Source: CAD feature listing. Evaluate the final solid. Frame: model axes, mm. Face numbers are marked on the shaded views. A direction names the side the tool comes from. Give positions to 0.01 mm unless a question says otherwise; leave off trailing zeros. Loops run counter-clockwise (first coordinate to the right, second up) from the corner with the lowest first, then second, coordinate; pieces in that order, holes last.
from build123d import *

# Parameters (mm, degrees)
SKETCH1_R                = 18.5
BOSS_EXTRUDE1_DEPTH      = 27.8
SKETCH2_R                = 17.1
BOSS_EXTRUDE2_DEPTH      = 25.2
SKETCH3_R                = 3.75
BOSS_EXTRUDE3_DEPTH      = 3.3
SKETCH4_R                = 6
BOSS_EXTRUDE4_DEPTH      = 6
SKETCH5_R                = 3
BOSS_EXTRUDE6_DEPTH      = 15
CUT_EXTRUDE1_START       = -12
CUT_EXTRUDE1_DEPTH       = 12
CUT_EXTRUDE2_DEPTH       = 1
M3_CLEARANCE_HOLE1_D     = 3.4
M3_CLEARANCE_HOLE1_DEPTH = 6
M3_CLEARANCE_HOLE1_TIP   = 1.021463052
SKETCH11_W               = 3
SKETCH11_H               = 0.5
BOSS_EXTRUDE7_DEPTH      = 8
FILLET1_R                = 1
CUT_EXTRUDE3_DEPTH       = 28


with BuildPart() as part:
    # Sketch1 → Boss-Extrude1 (new body)
    with BuildSketch(Plane.XY):
        Circle(SKETCH1_R)
    extrude(amount=BOSS_EXTRUDE1_DEPTH)

    # Sketch2 → Boss-Extrude2 (add)
    with BuildSketch(Plane(origin=(0, 0, 0), x_dir=(-1, 0, 0), z_dir=(0, 0, -1))):
        with Locations(Location((0, 0, 0), (0, 0, 180))):
            Circle(SKETCH2_R)
    extrude(amount=BOSS_EXTRUDE2_DEPTH)

    # Sketch3 → Boss-Extrude3 (add)
    with BuildSketch(Plane(origin=(0, 0, -25.2), x_dir=(-1, 0, 0), z_dir=(0, 0, -1))):
        Circle(SKETCH3_R)
    extrude(amount=BOSS_EXTRUDE3_DEPTH)

    # Sketch4 → Boss-Extrude4 (add)
    with BuildSketch(Plane.XY.offset(27.8)):
        with Locations((0, 7)):
            Circle(SKETCH4_R)
    extrude(amount=BOSS_EXTRUDE4_DEPTH)

    # Sketch5 → Boss-Extrude6 (add)
    with BuildSketch(Plane.XY.offset(33.8)):
        with Locations((0, 7)):
            Circle(SKETCH5_R)
    extrude(amount=BOSS_EXTRUDE6_DEPTH)

    # Sketch7 → Cut-Extrude1 (cut)
    with BuildSketch(Plane.XY.offset(48.8).offset(CUT_EXTRUDE1_START)):
        with BuildLine():
            Line((-1.8, 9.4), (1.8, 9.4))
            ThreePointArc((1.8, 9.4), (0, 10), (-1.8, 9.4))
        make_face()
    extrude(amount=CUT_EXTRUDE1_DEPTH, mode=Mode.SUBTRACT)

    # Sketch8 → Cut-Extrude2 (cut)
    with BuildSketch(Plane.XY.offset(27.8)):
        with BuildLine():
            ThreePointArc((8.923344727, 8.172142857), (0, -12.1), (-8.923344727, 8.172142857))
            ThreePointArc((-8.923344727, 8.172142857), (0, -2), (8.923344727, 8.172142857))
        make_face()
    extrude(amount=-CUT_EXTRUDE2_DEPTH, mode=Mode.SUBTRACT)

    # M3 Clearance Hole1
    with Locations(Plane.XY.offset(27.8)):
        with Locations((7.65, -13.250188678), (-7.65, -13.250188678), (-15.3, 0), (-7.65, 13.250188678), (15.3, 0), (7.65, 13.250188678)):
            Hole(M3_CLEARANCE_HOLE1_D / 2, depth=M3_CLEARANCE_HOLE1_DEPTH)
            with Locations((0, 0, -(M3_CLEARANCE_HOLE1_DEPTH + M3_CLEARANCE_HOLE1_TIP / 2))):  # 118° drill point
                Cone(0, M3_CLEARANCE_HOLE1_D / 2, M3_CLEARANCE_HOLE1_TIP, mode=Mode.SUBTRACT)

    # Sketch11 → Boss-Extrude7 (add)
    with BuildSketch(Plane(origin=(0, 0, -25.2), x_dir=(-1, 0, 0), z_dir=(0, 0, -1))):
        with Locations((0, 12)):
            Rectangle(SKETCH11_W, SKETCH11_H)
        with Locations((0, -12)):
            Rectangle(SKETCH11_W, SKETCH11_H)
    extrude(amount=BOSS_EXTRUDE7_DEPTH)

    # Fillet1
    fillet1_edges = [part.edges().sort_by_distance(p)[0] for p in [
        (-1.5, 12, -33.2),
        (1.5, 12, -33.2),
        (-1.5, -12, -33.2),
        (1.5, -12, -33.2),
    ]]
    fillet(fillet1_edges, radius=FILLET1_R)

    # Sketch12 → Cut-Extrude3 (cut)
    with BuildSketch(Plane(origin=(0, 12.25, 0), x_dir=(1, 0, 0), z_dir=(0, 1, 0))):
        with BuildLine():
            Line((0.492088327, 31.2), (0.492088327, 29.2))
            ThreePointArc((0.492088327, 29.2), (0, 28.707911673), (-0.492088327, 29.2))
            Line((-0.492088327, 29.2), (-0.492088327, 31.2))
            ThreePointArc((-0.492088327, 31.2), (0, 31.692088327), (0.492088327, 31.2))
        make_face()
    extrude(amount=-CUT_EXTRUDE3_DEPTH, mode=Mode.SUBTRACT)


solid = part.part
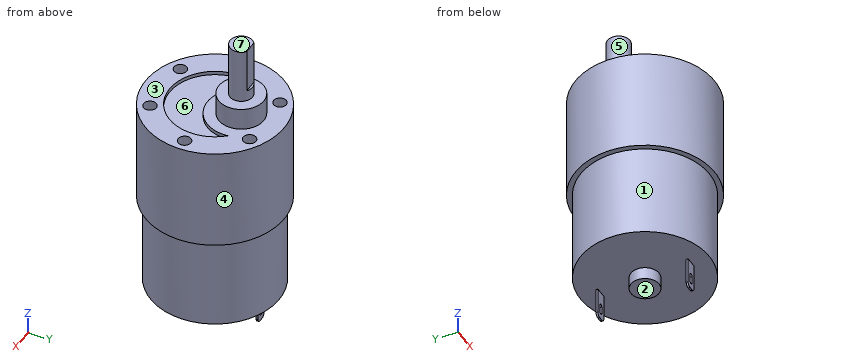
1) Cut plane C-C (x = 10.5). Return loops of the section in (y, z).
Checks:
outline: (-15.23, 0) - (-13.5, 0) - (-13.5, -25.2) - (13.5, -25.2) - (13.5, 0) - (15.23, 0) - (15.23, 27.8) - (6.01, 27.8) - (6.01, 26.8) - (-6.01, 26.8) - (-6.01, 27.8) - (-15.23, 27.8) - close
2) Cut plane B-B (y = 7). Return loops of the section in (x, z), and give its area (3 significant figures).
Checks:
outline: (-17.12, 0) - (-15.6, 0) - (-15.6, -25.2) - (15.6, -25.2) - (15.6, 0) - (17.12, 0) - (17.12, 27.8) - (9.87, 27.8) - (9.87, 26.8) - (9, 26.8) - (9, 27.8) - (6, 27.8) - (6, 33.8) - (3, 33.8) - (3, 48.8) - (-3, 48.8) - (-3, 33.8) - (-6, 33.8) - (-6, 27.8) - (-9, 27.8) - (-9, 26.8) - (-9.87, 26.8) - (-9.87, 27.8) - (-17.12, 27.8) - close
area: 1,900 mm2
3) Pull-direction query (Y, two-part tool) for the marked faces 5, 6 and 7; classes: released by +Y, released by -Y, zero draft, split by the parting line, or undercut.
Checks:
face 5: split by the parting line
face 6: undercut
face 7: zero draft
4) Reachability of the marked faces 1, 2, 3 and 4 from +Z, -Z, +X, -X, +Y, -Y: full face, straight path, thin tool, end or side. Return the list, or none.
Checks:
face 1: -Z
face 2: -Z, +X, -X
face 3: +Z
face 4: +Z, -Z
5) Contact query for flat-ended pins moving along their axis: P1, Ø4, axis at x = -1.5, z = 28, coming from the -Y side; P2, Ø3, axis at x = -7.65, y = 13.25, coming from the +Z side; P3, Ø0.6, axis at y = -12, z = -30, coming from the +X side. Output: stop coordinate, or through.
Checks:
P1: stops at y = -18.5
P2: stops at z = 21.68
P3: stops at x = 1.5
6) Ray query, probe 1 along Y at (x, z) = (-7.65, 24); probe 2 along Z at (x, y) = (-1, 8); probe 3 along Z at (x, y) = (9.5, 15.5). Return the intervals inside material, ascending.
Checks:
probe 1: y = -16.84 to -14.95, -11.55 to 11.55, 14.95 to 16.84
probe 2: z = -25.2 to 48.8
probe 3: z = 0 to 27.8
7) Cut plane A-A (z = 25). Return loops of the section in (x, y), and give its area (3 significant figures).
Checks:
outline: circle Ø37 at (0, 0); hole circle Ø3.4 at (-15.3, 0); hole circle Ø3.4 at (-7.65, -13.25); hole circle Ø3.4 at (-7.65, 13.25); hole circle Ø3.4 at (7.65, -13.25); hole circle Ø3.4 at (7.65, 13.25); hole circle Ø3.4 at (15.3, 0)
area: 1,020 mm2
8) Cut plane D-D (z = -13). Return loops of the section in (x, y).
Checks:
outline: circle Ø34.2 at (0, 0)
